```python
from build123d import *

# Parameters (mm, degrees)
SKETCH1_R           = 12.666666667
SKETCH1_R_2         = 45
BOSS_EXTRUDE1_DEPTH = 12
SKETCH2_R           = 57
SKETCH2_R_2         = 45
BOSS_EXTRUDE2_DEPTH = 51
SKETCH3_R           = 24.666666667
SKETCH3_R_2         = 12.666666667
BOSS_EXTRUDE3_DEPTH = 13
CUT_EXTRUDE1_DEPTH  = 3


with BuildPart() as part:
    # Sketch1 → Boss-Extrude1 (new body)
    with BuildSketch(Plane(origin=(0, 0, 0), x_dir=(1, 0, 0), z_dir=(0, 1, 0))):
        with BuildLine():
            Line((-19.4, 53.597014842), (-103.395321637, 23.194029815))
            ThreePointArc((-103.395321637, 23.194029815), (-119.666666667, 0), (-103.395321637, -23.194029815))
            Line((-103.395321637, -23.194029815), (-19.4, -53.597014842))
            ThreePointArc((-19.4, -53.597014842), (0, -57), (19.4, -53.597014842))
            Line((19.4, -53.597014842), (103.395321637, -23.194029815))
            ThreePointArc((103.395321637, -23.194029815), (119.666666667, 0), (103.395321637, 23.194029815))
            Line((103.395321637, 23.194029815), (19.4, 53.597014842))
            ThreePointArc((19.4, 53.597014842), (0, 57), (-19.4, 53.597014842))
        make_face()
        with Locations((-95, 0)):
            Circle(SKETCH1_R, mode=Mode.SUBTRACT)
        Circle(SKETCH1_R_2, mode=Mode.SUBTRACT)
        with Locations((95, 0)):
            Circle(SKETCH1_R, mode=Mode.SUBTRACT)
    extrude(amount=BOSS_EXTRUDE1_DEPTH)

    # Sketch2 → Boss-Extrude2 (add)
    with BuildSketch(Plane(origin=(0, 12, 0), x_dir=(1, 0, 0), z_dir=(0, 1, 0))):
        Circle(SKETCH2_R)
        Circle(SKETCH2_R_2, mode=Mode.SUBTRACT)
    extrude(amount=BOSS_EXTRUDE2_DEPTH)

    # Sketch3 → Boss-Extrude3 (add)
    with BuildSketch(Plane(origin=(0, 12, 0), x_dir=(1, 0, 0), z_dir=(0, 1, 0))):
        with Locations((95, 0)):
            Circle(SKETCH3_R)
        with Locations((95, 0)):
            Circle(SKETCH3_R_2, mode=Mode.SUBTRACT)
        with Locations((-95, 0)):
            Circle(SKETCH3_R)
        with Locations((-95, 0)):
            Circle(SKETCH3_R_2, mode=Mode.SUBTRACT)
    extrude(amount=BOSS_EXTRUDE3_DEPTH)

    # Sketch4 → Cut-Extrude1 (cut)
    with BuildSketch(Plane(origin=(0, 12, 0), x_dir=(1, 0, 0), z_dir=(0, 1, 0))):
        with BuildLine():
            Line((-42.970944355, 41.87478885), (-86.196761812, 26.228752198))
            ThreePointArc((-86.196761812, 26.228752198), (-67.333333333, 0), (-86.196761812, -26.228752198))
            Line((-86.196761812, -26.228752198), (-42.970944355, -41.87478885))
            ThreePointArc((-42.970944355, -41.87478885), (-60, 0), (-42.970944355, 41.87478885))
        make_face()
        with BuildLine():
            Line((38.798579703, -44.448511932), (89.505740572, -26.094524798))
            ThreePointArc((89.505740572, -26.094524798), (68.333333333, 0), (89.505740572, 26.094524798))
            Line((89.505740572, 26.094524798), (38.798579703, 44.448511932))
            ThreePointArc((38.798579703, 44.448511932), (59, 0), (38.798579703, -44.448511932))
        make_face()
    extrude(amount=-CUT_EXTRUDE1_DEPTH, mode=Mode.SUBTRACT)


solid = part.part
```
Check sheet for the modelled part. Datum: model origin and axes. Units: mm. A direction names the side the tool comes from. Coordinates: 2 decimals unless noted, no trailing zeros. Write each loop counter-clockwise with the first axis right and the second up, starting at its lowest first coordinate (ties: lowest second). Pieces come first, ordered by that corner, then holes. Notation, with made-up numbers: M 32,20 L 79,20 A13 ccw 79,43 Z; hole C 3,20 d5. An arc over 180 degrees is marked long. Write item = value, one per line. Start each with the question number.
1. Mould release check, pull along X, two halves, no side actions. Record for faces 4 (the flat face through (-61.99, 5.92, 38.18)), 5 (the flat face through (61.99, 5.92, -38.18)), 6 (the flat face through (106, 25, 11)), 7 (the flat face through (-64.28, 10.52, -34.16)): pulls with the +X half, pulls with the -X half, needs draft (parallel to the pull), parting line crosses it, or undercut.
2. Sectioned sample at D-D (x = -98). Record the cut outline in (y, z), then the cut area to 3 significant figures.
3. Tool access check on faces 1 (the flat face through (42, 63, -17)), 2 (the flat face through (-84, 25, 11)), 3 (the flat face through (-63, 9, 0)). Record the directions out of +Z, -Z, +X, -X, +Y, -Y that give a thin tool (end or side, any length) a straight path to the whole face; none if there is none.
4. Thickness scan on probe 1 along X at (y, z) = (10.75, 0); probe 2 along Z at (x, y) = (-95, 14.25); probe 3 along Z at (x, y) = (95, 6). Record the ranges inside material, lowest first.
5. Go/stop test with flat-tipped pins: pin 1 (5 mm diameter, centred on y = 16, z = 27.5, fed in from +X) (3 decimals); pin 2 (6 mm diameter, centred on x = 85, z = -30, fed in from +Y); pin 3 (10 mm diameter, centred on x = 53.5, y = 32.5, fed in from +Z). Record where each tip stops, or that it passes through.
6. Sectioned sample at A-A (x = 0). Record the cut outline in (y, z), then the cut area to 3 significant figures.
7. Sectioned sample at B-B (y = 54.5). Record the cut outline in (x, z).
8. Sectioned sample at C-C (x = 73.5). Record the cut outline in (y, z), then the cut area to 3 significant figures.
The answers:
q1.face_4 = pulls with the -X half
q1.face_5 = pulls with the +X half
q1.face_6 = needs draft
q1.face_7 = undercut
q2.outline = M 0,-25.15 L 12,-25.15 L 12,-24.48 L 25,-24.48 L 25,-12.31 L 0,-12.31 Z; M 0,12.31 L 25,12.31 L 25,24.48 L 12,24.48 L 12,25.15 L 0,25.15 Z
q2.area = 625 mm²
q3.face_1 = +Z, -Z, +X, -X, +Y
q3.face_2 = +Z, -Z, -X, +Y
q3.face_3 = +Y
q4.probe_1 = -119.67 to -107.67, -82.33 to -67.33, -60 to -45, 45 to 59, 68.33 to 82.33, 107.67 to 119.67
q4.probe_2 = -24.67 to -12.67, 12.67 to 24.67
q4.probe_3 = -26.23 to -12.67, 12.67 to 26.23
q5.pin_1 = 51.225
q5.pin_2 = 12
q5.pin_3 = 29.95
q6.outline = M 0,-57 L 63,-57 L 63,-45 L 0,-45 Z; M 0,45 L 63,45 L 63,57 L 0,57 Z
q6.area = 1,510 mm²
q7.outline = C 0,0 d114; hole C 0,0 d90
q8.outline = M 0,-34.01 L 12,-34.01 L 12,-31.89 L 9,-31.89 L 9,-15.78 L 12,-15.78 L 12,-12.09 L 25,-12.09 L 25,12.09 L 12,12.09 L 12,15.78 L 9,15.78 L 9,31.89 L 12,31.89 L 12,34.01 L 0,34.01 Z
q8.area = 1,030 mm²
